Read the model definition and answer for the solid it produces. Units are mm, in the model's axes. A direction names the side the tool comes from. Coordinates: 2 decimals unless noted, no trailing zeros. Write each loop counter-clockwise with the first axis right and the second up, starting at its lowest first coordinate (ties: lowest second). Pieces come first, ordered by that corner, then holes. Notation, with made-up numbers: M 38,-23.5 L 84,-23.5 A11 cw 84,-11.5 Z; hole C -26.5,49 d7. An arc over 180 degrees is marked long. Use a Markdown table: item, result. Add a question column.
Autodesk Inventor part; units mm, degrees
ref_plane "YZ Plane" through (0, 0, 0) normal (1, 0, 0) x (0, 1, 0)
ref_plane "XZ Plane" through (0, 0, 0) normal (0, 1, 0) x (-1, 0, 0)
ref_plane "XY Plane" through (0, 0, 0) normal (0, 0, 1) x (1, 0, 0)
sketch "Sketch1" plane through (0, 0, 0) normal (0, 0, 1) x (1, 0, 0)
  arc A0 (-25, 0) -> (0, 0) centre (-12.5, 0) ccw construction
  arc A1 (0, 0) -> (25, 0) centre (12.5, 0) ccw construction
  line L0 (-25, 0) -> (25, 0) construction
  line L1 (-25, 0) -> (-25, 4)
  line L2 (25, 0) -> (25, 4)
  arc A2 (-22.0802, 3.6444) -> (-2.9198, 3.6444) centre (-12.5, 0) ccw
  arc A3 (2.9198, 3.6444) -> (22.0802, 3.6444) centre (12.5, 0) ccw
  line L3 (-24, 5) -> (-23.0149, 5)
  line L4 (-1.9851, 5) -> (1.9851, 5)
  line L5 (23.0149, 5) -> (24, 5)
  arc A4 (2.4194, -7.3913) -> (-2.4194, -7.3913) centre (0, -9.1652) ccw
  arc A5 (-22.0802, 3.6444) -> (-23.0149, 5) centre (-23.0149, 4) ccw
  arc A6 (-24, 5) -> (-25, 4) centre (-24, 4) ccw
  arc A7 (-1.9851, 5) -> (-2.9198, 3.6444) centre (-1.9851, 4) ccw
  arc A8 (2.9198, 3.6444) -> (1.9851, 5) centre (1.9851, 4) ccw
  arc A9 (23.0149, 5) -> (22.0802, 3.6444) centre (23.0149, 4) ccw
  arc A10 (25, 4) -> (24, 5) centre (24, 4) ccw
  arc A11 (-25, 0) -> (-2.4194, -7.3913) centre (-12.5, 0) ccw
  arc A12 (2.4194, -7.3913) -> (25, 0) centre (12.5, 0) ccw
  line L6 (-24, 5) -> (-23.0149, 5)
  point P0 (25, 5)
  point P1 (-3.5522, 5)
  point P2 (3.5522, 5)
  point P3 (21.4478, 5)
  dimension "d0" = 12.5
  dimension "d2" = 12.5
  dimension "d3" = 5
  dimension "d5" = 10.25
  dimension "d6" = 10.25
  dimension "d9" = 3
  dimension "d10" = 1
  dimension "d11" = 1
extrude "Extrusion2" add sketch "Sketch1" along normal blind 60
equation "\"d2\" = d0"
equation "\"d6\" = d5"
properties part number "spool holder"
Item 1: Find section C-C on z = 33.5. Give the vertices of the cut face in (x, y).
Item 2: Find section B-B on y = -3.5. Give the vertices of the cut face in (x, z).
Item 3: Find section A-A on y = -8.5. Give the vertices of the cut face in (x, z), then the cut area to 3 significant figures.
Item 4: Determine the mould class of faces 3 (the flat face through (-25, 2, 30)), 4 (the flat face through (25, 2, 30)), 5 (the cylindrical face through (2.8, 4.58, 29.58)) for opening direction X: pulls with the +X half, pulls with the -X half, needs draft (parallel to the pull), parting line crosses it, or undercut.
Item 5: Find section D-D on x = -12.5. Give the vertices of the cut face in (y, z).
Item 6: For faces 1 (the flat face through (0, 5, 30)), 2 (the cylindrical face through (22.184, 4.556, 29.58)), determine the directions among +Z, -Z, +X, -X, +Y, -Y from which every point of the face is accessible in a straight line to the end or side of a thin tool.
Item 7: Each of these flat-tipped pins is pushed along its axis until it touches: pin 1 (5 mm diameter, centred on x = -6.5, z = 32.5, fed in from -Y); pin 2 (5 mm diameter, centred on x = 12.5, z = 40, fed in from +Y); pin 3 (10 mm diameter, centred on x = 12.5, z = 11.5, fed in from +Y). Where does it stop, or does it pass through?
Item 8: Consider probe 1 along X at (y, z) = (0, 25.5); probe 2 along X at (y, z) = (-4, 7); probe 3 along Y at (x, z) = (12, 35). Determine where each line is inside the solid, lowest interval first.
Geometry says:
| question | item | result |
|---|---|---|
| 1 | outline | M -25,0 A12.5 ccw -2.42,-7.39 A3 cw 2.42,-7.39 A12.5 ccw 25,0 L 25,4 A1 ccw 24,5 L 23.01,5 A1 ccw 22.08,3.64 A10.25 cw long 2.92,3.64 A1 ccw 1.99,5 L -1.99,5 A1 ccw -2.92,3.64 A10.25 cw long -22.08,3.64 A1 ccw -23.01,5 L -24,5 A1 ccw -25,4 Z |
| 2 | outline | M -24.5,0 L -22.13,0 L -22.13,60 L -24.5,60 Z; M -2.87,0 L 2.87,0 L 2.87,60 L -2.87,60 Z; M 22.13,0 L 24.5,0 L 24.5,60 L 22.13,60 Z |
| 3 | outline | M -21.67,0 L -18.23,0 L -18.23,60 L -21.67,60 Z; M -6.77,0 L -3.33,0 L -3.33,60 L -6.77,60 Z; M 3.33,0 L 6.77,0 L 6.77,60 L 3.33,60 Z; M 18.23,0 L 21.67,0 L 21.67,60 L 18.23,60 Z |
| 3 | area | 825 mm2 |
| 4 | face 3 | pulls with the -X half |
| 4 | face 4 | pulls with the +X half |
| 4 | face 5 | undercut |
| 5 | outline | M -12.5,0 L -10.25,0 L -10.25,60 L -12.5,60 Z |
| 6 | face 1 | +Z, -Z, +X, -X, +Y |
| 6 | face 2 | +Z, -Z |
| 7 | pin 1 | stops at y = -12 |
| 7 | pin 2 | stops at y = -9.94 |
| 7 | pin 3 | stops at y = -8.95 |
| 8 | probe 1 | x = -25 to -22.75, -2.25 to 2.25, 22.75 to 25 |
| 8 | probe 2 | x = -24.34 to -21.94, -3.06 to 3.06, 21.94 to 24.34 |
| 8 | probe 3 | y = -12.49 to -10.24 |
